For this review, take the finished solid that the model builds, in its own axes (mm). Face numbers are marked on the shaded views. A direction names the side the tool comes from. Round coordinates to 2 decimals unless told otherwise and drop trailing zeros. Write each loop counter-clockwise with the first axis right and the second up, starting at its lowest first coordinate (ties: lowest second). Pieces come first, ordered by that corner, then holes. Notation, with made-up numbers: M 41.25,57.5 L 87.25,57.5 A28 ccw 87.25,83.5 Z; hole C -33,78.5 d8. An arc over 180 degrees is marked long. Answer in a Markdown table with one row per item.
```python
from build123d import *

# Parameters (mm, degrees)
SKETCH1_R                      = 5
BASE_FLANGE1_DEPTH             = 3
EDGE_FLANGE1_STRIP_W           = 18
EDGE_FLANGE1_STRIP_H           = 3
EDGE_FLANGE1_STRIP_CUT_DEPTH   = 100
EDGE_FLANGE1_STRIP_2_W         = 18
EDGE_FLANGE1_STRIP_2_H         = 3
EDGE_FLANGE1_STRIP_CUT_2_DEPTH = 100
EDGE_FLANGE1_DEPTH             = 100
EDGE_FLANGE1_BEND_DEPTH        = 100
EDGE_FLANGE2_STRIP_W           = 18
EDGE_FLANGE2_STRIP_H           = 3
EDGE_FLANGE2_STRIP_CUT_DEPTH   = 100
EDGE_FLANGE2_STRIP_2_W         = 18
EDGE_FLANGE2_STRIP_2_H         = 3
EDGE_FLANGE2_STRIP_CUT_2_DEPTH = 100
EDGE_FLANGE2_DEPTH             = 100
EDGE_FLANGE2_BEND_DEPTH        = 100
SKETCHED_START                 = 58
SKETCHED_BEND1_OUTLINE_W       = 20
SKETCHED_BEND1_OUTLINE_H       = 3
SKETCHED_BEND1_DEPTH           = 33
SKETCHED_START_2               = 55
SKETCHED_BEND1_2_OUTLINE_R     = 5
SKETCHED_BEND1_2_DEPTH         = 3
SKETCHED_START_3               = -11
SKETCHED_BEND1_3_DEPTH         = 22


with BuildPart() as part:
    # Base-Flange1: sheet metal written as solids
    # Sketch1 → Base-Flange1 (new body)
    with BuildSketch(Plane(origin=(0, 0, 0), x_dir=(1, 0, 0), z_dir=(0, 1, 0))):
        with BuildLine():
            Line((10, 50), (10, 80))
            ThreePointArc((10, 80), (0, 90), (-10, 80))
            Line((-10, 80), (-10, 50))
            Line((-10, 50), (-50, 50))
            Line((-50, 50), (-50, -50))
            Line((-50, -50), (-10, -50))
            Line((-10, -50), (-10, -80))
            ThreePointArc((-10, -80), (0, -90), (10, -80))
            Line((10, -80), (10, -50))
            Line((10, -50), (50, -50))
            Line((50, -50), (50, 50))
            Line((50, 50), (10, 50))
        make_face()
        with Locations(Location((0, 80, 0), (0, 0, 270))):
            Circle(SKETCH1_R, mode=Mode.SUBTRACT)
        with Locations(Location((0, -80, 0), (0, 0, 90))):
            Circle(SKETCH1_R, mode=Mode.SUBTRACT)
    extrude(amount=-BASE_FLANGE1_DEPTH)

    # Edge-Flange1: sheet metal written as solids
    # Edge-Flange1 strip (on a plane across the edge) → Edge-Flange1 strip cut (cut)
    with BuildSketch(Plane(origin=(50, 0, 50), x_dir=(-1, 0, 0), z_dir=(0, 0, -1))):
        with Locations((-3, -1.5)):
            Rectangle(EDGE_FLANGE1_STRIP_W, EDGE_FLANGE1_STRIP_H)
    extrude(amount=EDGE_FLANGE1_STRIP_CUT_DEPTH, mode=Mode.SUBTRACT)

    # Edge-Flange1 strip 2 (on a plane across the edge) → Edge-Flange1 strip cut 2 (cut)
    with BuildSketch(Plane(origin=(-50, 0, -50), x_dir=(1, 0, 0), z_dir=(0, 0, 1))):
        with Locations((-3, -1.5)):
            Rectangle(EDGE_FLANGE1_STRIP_2_W, EDGE_FLANGE1_STRIP_2_H)
    extrude(amount=EDGE_FLANGE1_STRIP_CUT_2_DEPTH, mode=Mode.SUBTRACT)

    # Edge-Flange1 section (on a plane across the edge) → Edge-Flange1 (add)
    with BuildSketch(Plane(origin=(50, 0, 50), x_dir=(-1, 0, 0), z_dir=(0, 0, -1))):
        with BuildLine():
            Line((0, 3), (0, 37))
            Line((0, 37), (3, 37))
            Line((3, 37), (3, 3))
            ThreePointArc((3, 3), (3.878679656, 0.878679656), (6, 0))
            Line((6, 0), (6, -3))
            ThreePointArc((6, -3), (1.757359313, -1.242640687), (0, 3))
        make_face()
    extrude(amount=EDGE_FLANGE1_DEPTH)

    # Edge-Flange1 section 2 (on a plane across the edge) → Edge-Flange1 bend (add)
    with BuildSketch(Plane(origin=(-50, 0, -50), x_dir=(1, 0, 0), z_dir=(0, 0, 1))):
        with BuildLine():
            Line((0, 3), (0, 37))
            Line((0, 37), (3, 37))
            Line((3, 37), (3, 3))
            ThreePointArc((3, 3), (3.878679656, 0.878679656), (6, 0))
            Line((6, 0), (6, -3))
            ThreePointArc((6, -3), (1.757359313, -1.242640687), (0, 3))
        make_face()
    extrude(amount=EDGE_FLANGE1_BEND_DEPTH)

    # Edge-Flange2: sheet metal written as solids
    # Edge-Flange2 strip (on a plane across the edge) → Edge-Flange2 strip cut (cut)
    with BuildSketch(Plane(origin=(-50, 37, 50), x_dir=(0, -1, 0), z_dir=(0, 0, -1))):
        with Locations((-6, -1.5)):
            Rectangle(EDGE_FLANGE2_STRIP_W, EDGE_FLANGE2_STRIP_H)
    extrude(amount=EDGE_FLANGE2_STRIP_CUT_DEPTH, mode=Mode.SUBTRACT)

    # Edge-Flange2 strip 2 (on a plane across the edge) → Edge-Flange2 strip cut 2 (cut)
    with BuildSketch(Plane(origin=(50, 37, -50), x_dir=(0, -1, 0), z_dir=(0, 0, 1))):
        with Locations((-6, -1.5)):
            Rectangle(EDGE_FLANGE2_STRIP_2_W, EDGE_FLANGE2_STRIP_2_H)
    extrude(amount=EDGE_FLANGE2_STRIP_CUT_2_DEPTH, mode=Mode.SUBTRACT)

    # Edge-Flange2 section (on a plane across the edge) → Edge-Flange2 (add)
    with BuildSketch(Plane(origin=(-50, 37, 50), x_dir=(0, -1, 0), z_dir=(0, 0, -1))):
        with BuildLine():
            Line((-3, 3), (-3, 25))
            Line((-3, 25), (0, 25))
            Line((0, 25), (0, 3))
            ThreePointArc((0, 3), (0.878679656, 0.878679656), (3, 0))
            Line((3, 0), (3, -3))
            ThreePointArc((3, -3), (-1.242640687, -1.242640687), (-3, 3))
        make_face()
    extrude(amount=EDGE_FLANGE2_DEPTH)

    # Edge-Flange2 section 2 (on a plane across the edge) → Edge-Flange2 bend (add)
    with BuildSketch(Plane(origin=(50, 37, -50), x_dir=(0, -1, 0), z_dir=(0, 0, 1))):
        with BuildLine():
            Line((-3, 3), (-3, 25))
            Line((-3, 25), (0, 25))
            Line((0, 25), (0, 3))
            ThreePointArc((0, 3), (0.878679656, 0.878679656), (3, 0))
            Line((3, 0), (3, -3))
            ThreePointArc((3, -3), (-1.242640687, -1.242640687), (-3, 3))
        make_face()
    extrude(amount=EDGE_FLANGE2_BEND_DEPTH)

    # Sketched Bend1: read off the stored shape, not the designer's step
    # Sketched Bend1 outline → Sketched Bend1 (cut)
    with BuildSketch(Plane.XY.offset(SKETCHED_START)):
        with Locations((0, -1.5)):
            Rectangle(SKETCHED_BEND1_OUTLINE_W, SKETCHED_BEND1_OUTLINE_H)
    extrude(amount=SKETCHED_BEND1_DEPTH, mode=Mode.SUBTRACT)

    # Sketched Bend1 2 outline → Sketched Bend1 2 (add)
    with BuildSketch(Plane.XY.offset(SKETCHED_START_2)):
        with BuildLine():
            ThreePointArc((10, 22.64380551), (0, 32.64380551), (-10, 22.64380551))
            Line((-10, 22.64380551), (-10, 0))
            Line((-10, 0), (10, 0))
            Line((10, 0), (10, 22.64380551))
        make_face()
        with Locations((0, 22.64380551)):
            Circle(SKETCHED_BEND1_2_OUTLINE_R, mode=Mode.SUBTRACT)
    extrude(amount=SKETCHED_BEND1_2_DEPTH)

    # Sketched Bend1 3 outline → Sketched Bend1 3 (cut)
    with BuildSketch(Plane.YZ.offset(SKETCHED_START_3)):
        with BuildLine():
            ThreePointArc((-3, 55), (-2.121320344, 57.121320344), (0, 58))
            Line((0, 58), (-3, 58))
            Line((-3, 58), (-3, 55))
        make_face()
    extrude(amount=SKETCHED_BEND1_3_DEPTH, mode=Mode.SUBTRACT)


solid = part.part
```
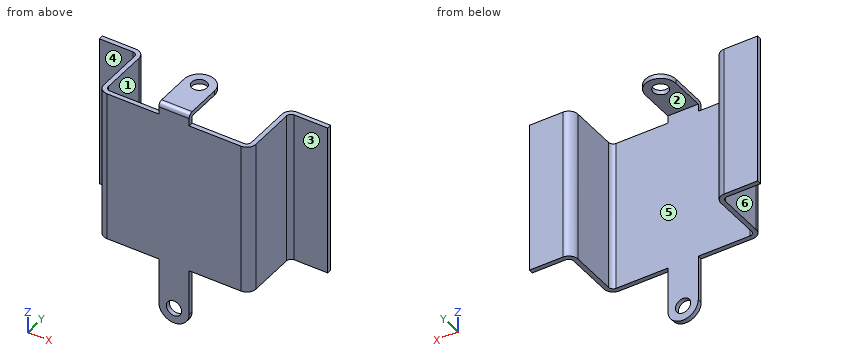
Q1. For probe 1 along X at (y, z) = (26.5, 24); probe 2 along X at (y, z) = (-1, -80); probe 3 along Z at (x, y) = (48, 11.5), list the stretches that pass through material, from the lowest coordinate up.
Found:
| item | result |
|---|---|
| probe 1 | -50 to -47, 47 to 50 |
| probe 2 | -10 to -5, 5 to 10 |
| probe 3 | -50 to 50 |
Q2. Machinability: for the marked faces 1, 2 and 3, which of the approach directions +Z, -Z, +X, -X, +Y, -Y give a long, thin tool a straight path to every point of the face, cutting with its end or side? Answer none if there is none.
Found:
| item | result |
|---|---|
| face 1 | +Z, -Z, +Y |
| face 2 | -Z, +X, -X, +Y |
| face 3 | +Z, -Z, +X, -Y |
Q3. Insertion check: P1, Ø4, axis at x = -21, z = -33, coming from the +Y side; P2, Ø9, axis at x = 0, y = 22.64, coming from the -Z side; P3, Ø5, axis at x = -58.5, z = 15.5, coming from the -Y side; P4, Ø12, axis at y = 7, z = 20, coming from the -X side. Each pin has a flat end and moves straight along its axis. Give the tip position at first contact, or say it passes through.
Found:
| item | result |
|---|---|
| P1 | y = 0 |
| P2 | through |
| P3 | y = 37 |
| P4 | x = -50 |
Q4. Mouldability with a two-part tool opening along X and no side actions: class the marked faces 4, 5 and 6 as +X half, -X half, draft (parallel to the pull), parting line (faces both ways), or undercut.
Found:
| item | result |
|---|---|
| face 4 | draft |
| face 5 | undercut |
| face 6 | -X half |
Q5. Take a section at B-B (y = 15.5). State the section outline as (x, z) points, then the cut area to 3 significant figures.
Found:
| item | result |
|---|---|
| outline | M -50,-50 L -47,-50 L -47,50 L -50,50 Z; M -10,55 L 10,55 L 10,58 L -10,58 Z; M 47,-50 L 50,-50 L 50,50 L 47,50 Z |
| area | 660 mm² |
Q6. Take a section at D-D (x = 56.5). State the section outline as (y, z) points, then the cut area to 3 significant figures.
Found:
| item | result |
|---|---|
| outline | M 37,-50 L 40,-50 L 40,50 L 37,50 Z |
| area | 300 mm² |
Q7. Take a section at A-A (x = 0). State the section outline as (y, z) points, then the cut area to 3 significant figures.
Found:
| item | result |
|---|---|
| outline | M -3,-90 L 0,-90 L 0,-85 L -3,-85 Z; M -3,-75 L 0,-75 L 0,55 L 17.64,55 L 17.64,58 L 0,58 A3 ccw -3,55 Z; M 27.64,55 L 32.64,55 L 32.64,58 L 27.64,58 Z |
| area | 480 mm² |
Q8. Take a section at C-C (z = 9). State the section outline as (x, y) points.
Found:
| item | result |
|---|---|
| outline | M -75,37 L -53,37 A3 cw -50,34 L -50,3 A6 ccw -44,-3 L 44,-3 A6 ccw 50,3 L 50,34 A3 cw 53,37 L 75,37 L 75,40 L 53,40 A6 ccw 47,34 L 47,3 A3 cw 44,0 L -44,0 A3 cw -47,3 L -47,34 A6 ccw -53,40 L -75,40 Z |
